Job drawing, mm, ordinate dimensions from the low corner. One solid piece. A direction names the side the tool comes from. Give positions to 0.01 mm unless a question says otherwise; leave off trailing zeros. Loops run counter-clockwise (first coordinate to the right, second up) from the corner with the lowest first, then second, coordinate; pieces in that order, holes last.
Item 1: Saw through at A-A on x = 67.31. Give the number of separate pieces and of enclosed holes in the cut face, plus the area to 3 significant figures.
Item 2: Drop flat-ended pins along their axis: P1, Ø3, axis at y = 17.5, z = 40.5, coming from the +X side; P2, Ø8, axis at x = 38.02, y = 18.18, coming from the -Z side; P3, Ø1.1, axis at y = 17.5, z = 40, coming from the -X side; P4, Ø2, axis at x = 19, y = 8.5, coming from the +Z side. Give the stop position or say it passes through.
Item 3: Saw through at C-C on y = 33. Give the cut face in (x, z) (1 decimal).
Item 4: Mould opens along Y. For the marked faces 3, 4 and 5 say: released by +Y, released by -Y, zero draft, split by the parting line, or undercut.
Item 5: Probe probe 1 along Y at (x, z) = (8.89, 19.5); probe 2 along X at (y, z) = (6, 17) (1 decimal); probe 3 along Z at (x, y) = (35.5, 23). List the from-to ranges inside material, lowest first.
Item 6: Which spindle directions (+Z, -Z, +X, -X, +Y, -Y) get a long thin tool onto all of the face, cutting with end or side? Do the marked faces 1 and 2. Say none if no direction does.
Item 7: Saw through at B-B on z = 21.5. Give the cut face in (x, y).
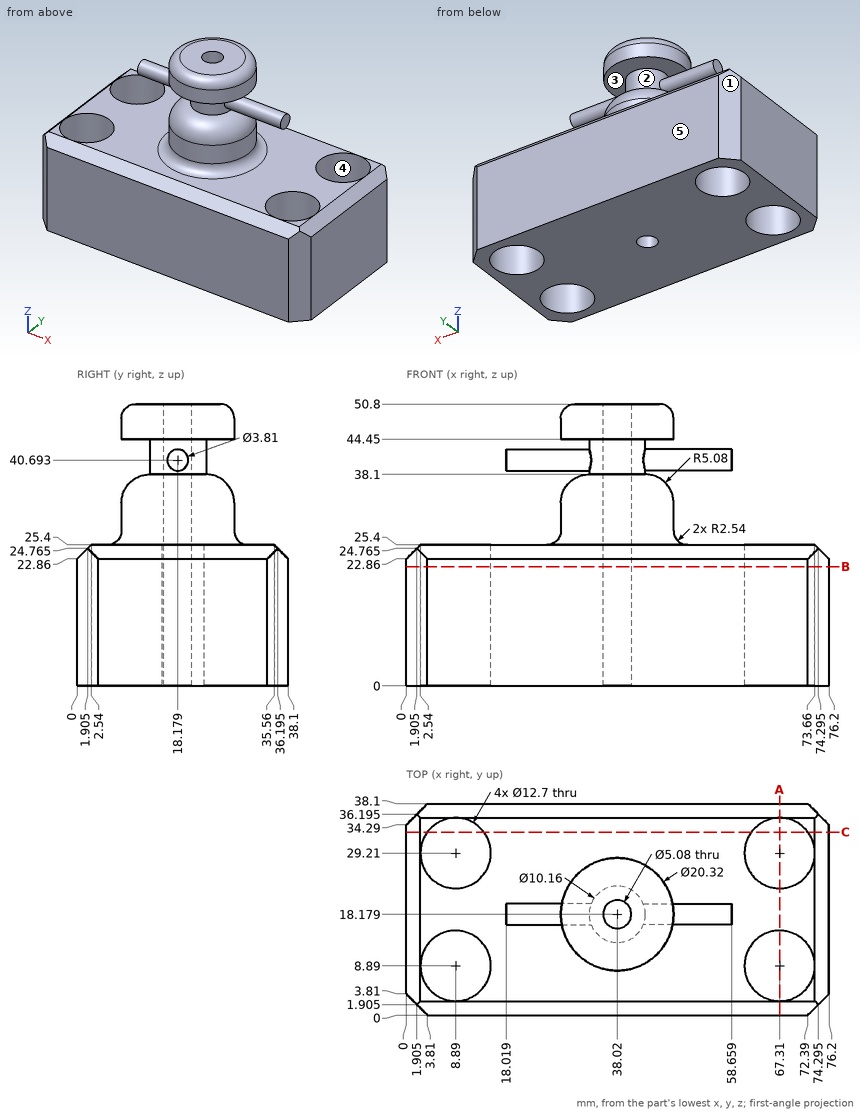
Results below:
1. separate pieces: 3
1. enclosed holes: 0
1. area: 316 mm2
2. P1: stops at x = 58.66
2. P2: stops at z = 0
2. P3: stops at x = 18.02
2. P4: stops at z = 25.4
3. outline: (0, 0) - (3.8, 0) - (3.8, 25.4) - (2.5, 25.4) - (0, 22.9) - close; (14, 0) - (62.2, 0) - (62.2, 25.4) - (14, 25.4) - close; (72.4, 0) - (76.2, 0) - (76.2, 22.9) - (73.7, 25.4) - (72.4, 25.4) - close
4. face 3: zero draft
4. face 4: undercut
4. face 5: released by +Y
5. probe 1: y = 0 to 2.54, 15.24 to 22.86, 35.56 to 38.1
5. probe 2: x = 0 to 3.2, 14.5 to 61.7, 73 to 76.2
5. probe 3: z = 0 to 38.09, 44.45 to 50.8
6. face 1: +Z, -Z, -X, +Y
6. face 2: none
7. outline: (0, 3.81) - (3.81, 0) - (72.39, 0) - (76.2, 3.81) - (76.2, 34.29) - (72.39, 38.1) - (3.81, 38.1) - (0, 34.29) - close; hole circle Ø12.7 at (8.89, 8.89); hole circle Ø12.7 at (8.89, 29.21); hole circle Ø5.08 at (38.02, 18.18); hole circle Ø12.7 at (67.31, 8.89); hole circle Ø12.7 at (67.31, 29.21)
